```python
from build123d import *

# Parameters (mm, degrees)
SKETCH1_R           = 27.5
SKETCH1_R_2         = 2.5
SKETCH1_R_3         = 3.25
BOSS_EXTRUDE1_DEPTH = 3.1


with BuildPart() as part:
    # Sketch1 → Boss-Extrude1 (new body)
    with BuildSketch(Plane.XY):
        Circle(SKETCH1_R)
        with Locations((-6.914797213, 6.914797213)):
            Circle(SKETCH1_R_2, mode=Mode.SUBTRACT)
        with Locations((6.914797213, 6.914797213)):
            Circle(SKETCH1_R_2, mode=Mode.SUBTRACT)
        with Locations((6.914797213, -6.914797213)):
            Circle(SKETCH1_R_2, mode=Mode.SUBTRACT)
        with Locations((-6.914797213, -6.914797213)):
            Circle(SKETCH1_R_2, mode=Mode.SUBTRACT)
        with Locations((15.0260191, -15.0260191)):
            Circle(SKETCH1_R_3, mode=Mode.SUBTRACT)
        with Locations((-15.0260191, -15.0260191)):
            Circle(SKETCH1_R_3, mode=Mode.SUBTRACT)
        with Locations((-15.0260191, 15.0260191)):
            Circle(SKETCH1_R_3, mode=Mode.SUBTRACT)
        with Locations((15.0260191, 15.0260191)):
            Circle(SKETCH1_R_3, mode=Mode.SUBTRACT)
        with Locations((0, -15)):
            Circle(SKETCH1_R_3, mode=Mode.SUBTRACT)
        with Locations((0, 15)):
            Circle(SKETCH1_R_3, mode=Mode.SUBTRACT)
    extrude(amount=BOSS_EXTRUDE1_DEPTH)


solid = part.part
```
Here's how the part is built. I have some questions about the finished solid (model axes, mm). Coordinates: 2 decimals unless noted, no trailing zeros. Write each loop counter-clockwise with the first axis right and the second up, starting at its lowest first coordinate (ties: lowest second). Pieces come first, ordered by that corner, then holes. Notation, with made-up numbers: (-12.5, -4.5) - (13.5, -4.5) arc R19 ccw to (13.5, 26.5) - close; hole circle Ø4 at (18.5, -6.75). An arc over 180 degrees is marked (long way). One line per item, written item: value.
1) I need wall thicknesses on line 1 along Y through (x, z) = (0, 1.75); line 2 along X through (y, z) = (13.5, 2.6); line 3 along X through (y, z) = (-18, 0.3). Which ranges of each line are inside material? Lowest first, please.
Model answer:
line 1: y = -27.5 to -18.25, -11.75 to 11.75, 18.25 to 27.5
line 2: x = -23.96 to -17.9, -12.16 to -2.88, 2.88 to 12.16, 17.9 to 23.96
line 3: x = -20.79 to -16.34, -13.72 to -1.25, 1.25 to 13.72, 16.34 to 20.79
2) Suppose I cut it at A-A on x = 0. Write out the boundary of the cut face in (y, z), and give its area (3 significant figures).
Model answer:
outline: (-27.5, 0) - (-18.25, 0) - (-18.25, 3.1) - (-27.5, 3.1) - close; (-11.75, 0) - (11.75, 0) - (11.75, 3.1) - (-11.75, 3.1) - close; (18.25, 0) - (27.5, 0) - (27.5, 3.1) - (18.25, 3.1) - close
area: 130 mm²
3) We'd pull the mould along X, two halves only. Please class faces 1 (the flat face through (0, 0, 0)), 2 (the cylindrical face through (-0.423, 18.222, 1.528)), 3 (the cylindrical face through (-5.961, -26.846, 1.528)): pulls with the +X half, pulls with the -X half, needs draft (parallel to the pull), parting line crosses it, or undercut.
Model answer:
face 1: needs draft
face 2: undercut
face 3: parting line crosses it
4) Suppose I cut it at B-B on z = 2.3. State how many separate pieces and enclosed holes the cut face has, and give its area (3 significant figures).
Model answer:
separate pieces: 1
enclosed holes: 10
area: 2,100 mm²
5) I'm going to push flat-ended pins straight in: P1, Ø4, axis at x = 15.03, y = 15.03, coming from the -Z side; P2, Ø1, axis at y = 20.5, z = 1, coming from the +X side; P3, Ø1.5, axis at x = -12.5, z = 1.5, coming from the +Y side. Where does each tip first touch, or does it pass through?
Model answer:
P1: passes through
P2: stops at x = 18.87
P3: stops at y = 24.86
6) Suppose I cut it at C-C on x = -16. Write out the boundary of the cut face in (y, z), and give its area (3 significant figures).
Model answer:
outline: (-22.37, 0) - (-18.13, 0) - (-18.13, 3.1) - (-22.37, 3.1) - close; (-11.93, 0) - (11.93, 0) - (11.93, 3.1) - (-11.93, 3.1) - close; (18.13, 0) - (22.37, 0) - (22.37, 3.1) - (18.13, 3.1) - close
area: 100 mm²
7) Suppose I cut it at D-D on y = 11. Write out the boundary of the cut face in (x, z).
Model answer:
outline: (-25.2, 0) - (25.2, 0) - (25.2, 3.1) - (-25.2, 3.1) - close
